from build123d import *

# Parameters (mm, degrees)
SKETCH1_R           = 13.97
SKETCH1_R_2         = 8.5
BOSS_EXTRUDE1_DEPTH = 12.7
FILLET1_R           = 0.5


with BuildPart() as part:
    # Sketch1 → Boss-Extrude1 (new body)
    with BuildSketch(Plane.XY):
        Circle(SKETCH1_R)
        Circle(SKETCH1_R_2, mode=Mode.SUBTRACT)
    extrude(amount=BOSS_EXTRUDE1_DEPTH)

    # Fillet1
    fillet1_edges = [part.edges().sort_by_distance(p)[0] for p in [
        (-13.97, 0, 0),
        (-13.97, 0, 12.7),
    ]]
    fillet(fillet1_edges, radius=FILLET1_R)

    # Sketch2 → Revolve1 (revolve)
    with BuildSketch(Plane(origin=(0, 0, 0), x_dir=(0, 0, -1), z_dir=(1, 0, 0))):
        Polygon((0, 8.5), (-12.7, 8.5), (-12.7, 9.5), (-13.2, 9.5), (-13.2, 8), (-4, 8), (-4, 1.5), (0.5, 1.5), (0.5, 9.5), (0, 9.5), align=None)
    revolve(axis=Axis((0, 0, 0), (0, 0, 1)))


solid = part.part
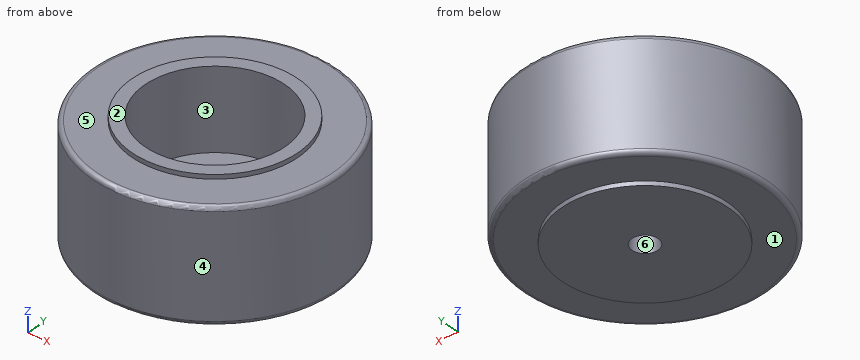
Check sheet for the modelled part. Datum: model origin and axes. Units: mm. Face numbers are marked on the shaded views. A direction names the side the tool comes from. Give positions to 0.01 mm unless a question says otherwise; leave off trailing zeros. Write each loop counter-clockwise with the first axis right and the second up, starting at its lowest first coordinate (ties: lowest second). Pieces come first, ordered by that corner, then holes. Notation, with made-up numbers: (63.25, 86.5) -> (77.25, 86.5) arc R24 ccw to (77.25, 113.5) -> close; hole circle Ø7 at (-27, -32). An arc over 180 degrees is marked (long way). One line per item, written item: value. Start each with the question number.
Item 1: Gauge pin test, flat ends, axial feed: pin 1 (2 mm diameter, centred on x = -2.5, z = 2, fed in from -Y); pin 2 (8 mm diameter, centred on y = 0.5, z = 5, fed in from -X); pin 3 (1 mm diameter, centred on x = -2, z = 10.5, fed in from +Y); pin 4 (8 mm diameter, centred on y = -9.5, z = 4.5, fed in from +X). Record the tip position at first contact, or that the pin passes through.
Item 2: Section check C-C on z = 2.5. Record the cut outline in (x, y), then the cut area to 3 significant figures.
Item 3: Material ranges on probe 1 along Y at (x, z) = (0, 11); probe 2 along Y at (x, z) = (0, 1.1); probe 3 along Z at (x, y) = (-5.25, -5.5), recorded low to high. Write a range as from..to.
Item 4: Section check D-D on z = 6. Record the cut outline in (x, y).
Item 5: Draft check along X on the marked faces 3, 4, 5 and 6. Enter one of: +X half, -X half, draft (parallel to the pull), parting line (faces both ways), or undercut.
Item 6: Section check A-A on x = 0. Record the cut outline in (y, z).
Item 7: Tool access check on the marked faces 1 and 2. Record the directions out of +Z, -Z, +X, -X, +Y, -Y that give a thin tool (end or side, any length) a straight path to the whole face; none if there is none.
Results list:
1. pin 1: y = -13.89
1. pin 2: x = -13.97
1. pin 3: y = 13.89
1. pin 4: x = 12.84
2. outline: circle Ø27.94 at (0, 0); hole circle Ø3 at (0, 0)
2. area: 606 mm²
3. probe 1: -13.97..-8, 8..13.97
3. probe 2: -13.97..-1.5, 1.5..13.97
3. probe 3: -0.5..4
4. outline: circle Ø27.94 at (0, 0); hole circle Ø16 at (0, 0)
5. face 3: undercut
5. face 4: parting line
5. face 5: draft
5. face 6: undercut
6. outline: (-13.97, 0.5) arc R0.5 ccw to (-13.47, 0) -> (-9.5, 0) -> (-9.5, -0.5) -> (-1.5, -0.5) -> (-1.5, 4) -> (-8, 4) -> (-8, 13.2) -> (-9.5, 13.2) -> (-9.5, 12.7) -> (-13.47, 12.7) arc R0.5 ccw to (-13.97, 12.2) -> close; (1.5, -0.5) -> (9.5, -0.5) -> (9.5, 0) -> (13.47, 0) arc R0.5 ccw to (13.97, 0.5) -> (13.97, 12.2) arc R0.5 ccw to (13.47, 12.7) -> (9.5, 12.7) -> (9.5, 13.2) -> (8, 13.2) -> (8, 4) -> (1.5, 4) -> close
7. face 1: -Z
7. face 2: +Z, +X, -X, +Y, -Y
